```python
from build123d import *

# Parameters (mm, degrees)
F1_DEPTH = 2
F2_DEPTH = 27
F4_DEPTH = 25


with BuildPart() as f1:
    # F0 (on Top) → F1 (new body)
    with BuildSketch(Plane.XY):
        Polygon((-45, -24.5), (45, -24.5), (45, -22.5), (45, 22.5), (-45, 22.5), (-45, -22.5), align=None)
    extrude(amount=F1_DEPTH)

    # F0 (on Top) → F2 (join)
    with BuildSketch(Plane.XY):
        Polygon((47, -24.5), (47, 24.5), (-47, 24.5), (-47, -24.5), (-45, -24.5), (-45, -22.5), (-45, 22.5), (45, 22.5), (45, -22.5), (45, -24.5), align=None)
    extrude(amount=F2_DEPTH)

    # F3 (on face) → F4 (cut)
    with BuildSketch(Plane(origin=(0, 24.5, 0), x_dir=(-1, 0, 0), z_dir=(0, 1, 0))):
        with BuildLine():
            Line((39.115214, 27), (-39.115214, 27))
            ThreePointArc((-39.115214, 27), (0, 9), (39.115214, 27))
        make_face()
    extrude(amount=-F4_DEPTH, mode=Mode.SUBTRACT)


solid = f1.part
```
Input: part model. Units: mm. Frame: model coordinates. A direction names the side the tool comes from. Give positions to 0.01 mm unless a question says otherwise; leave off trailing zeros. Order: outer loops, then holes, each group sorted by start corner. A loop starts at its lowest first (then second) coordinate and runs counter-clockwise, first axis right, second up. Notation, with made-up numbers: (-8.75, 53.25) - (23.25, 53.25) arc R15 ccw to (23.25, 79.25) - close; hole circle Ø7 at (39, -17). An arc over 180 degrees is marked (long way). Use a Markdown table: item, result.
(1) Section query B-B (y = -12.5). Output: boundary loops of the cut face in (x, z).
Computed values:
| item | result |
|---|---|
| outline | (-47, 0) - (47, 0) - (47, 27) - (45, 27) - (45, 2) - (-45, 2) - (-45, 27) - (-47, 27) - close |
(2) Line query: line 1 (X direction, y = 6.5, z = 24.75); line 2 (Z direction, x = -28, y = 14); line 3 (Y direction, x = 37, z = 13.5). Output: solid intervals per line, ascending. Write a range as from..to.
Computed values:
| item | result |
|---|---|
| line 1 | x = -47..-45, 45..47 |
| line 2 | z = 0..2 |
| line 3 | y = 22.5..24.5 |
(3) Section query A-A (z = 24.25). Output: boundary loops of the cut face in (x, y), then the cut area to 3 significant figures.
Computed values:
| item | result |
|---|---|
| outline | (-47, -24.5) - (-45, -24.5) - (-45, 22.5) - (-36.58, 22.5) - (-36.58, 24.5) - (-47, 24.5) - close; (36.58, 22.5) - (45, 22.5) - (45, -24.5) - (47, -24.5) - (47, 24.5) - (36.58, 24.5) - close |
| area | 230 mm2 |
(4) Pin query (flat end, axial travel): pin 1 (1.5 mm diameter, centred on x = 5, y = 0, fed in from -Z); pin 2 (12 mm diameter, centred on x = -25, z = 14.5, fed in from -Y); pin 3 (5 mm diameter, centred on x = -33.5, y = -17, fed in from +Z). Return the tip coordinate at first contact, or that it passes through.
Computed values:
| item | result |
|---|---|
| pin 1 | stops at z = 0 |
| pin 2 | stops at y = 22.5 |
| pin 3 | stops at z = 2 |
(5) Access query for faces 1 (the flat face through (-0.6, 22.5, 8.8)), 2 (the flat face through (-4, -24.5, 1)). Directions: +Z, -Z, +X, -X, +Y, -Y. A direction counts if a zero-diameter tool reaches every point of the face in a straight line with its end or side. Return the directions, or none.
Computed values:
| item | result |
|---|---|
| face 1 | +Z, -Y |
| face 2 | +Z, -Z, +X, -X, -Y |
(6) Section query D-D (x = 26.5). Output: boundary loops of the cut face in (y, z), then the cut area to 3 significant figures.
Computed values:
| item | result |
|---|---|
| outline | (-24.5, 0) - (24.5, 0) - (24.5, 16.34) - (22.5, 16.34) - (22.5, 2) - (-24.5, 2) - close |
| area | 127 mm2 |
(7) Section query C-C (z = 8). Output: boundary loops of the cut face in (x, y), then the cut area to 3 significant figures.
Computed values:
| item | result |
|---|---|
| outline | (-47, -24.5) - (-45, -24.5) - (-45, 22.5) - (45, 22.5) - (45, -24.5) - (47, -24.5) - (47, 24.5) - (-47, 24.5) - close |
| area | 376 mm2 |
